from build123d import *

# Parameters (mm, degrees)
F0_W     = 30
F0_H     = 45
F1_DEPTH = 2
F2_W     = 30
F2_H     = 2
F2_H_2   = 5.5
F3_DEPTH = 2
F6_DEPTH = 25
F7_W     = 8
F7_H     = 11
F8_DEPTH = 2
F9_R     = 15
F10_R    = 5
F11_R    = 0.99999


# Not quite as in the source:
# - a fillet or chamfer is up to 0.001 mm smaller than in the source, because OpenCascade refuses the exact size
# - ends of sketch curves that miss each other by under 0.0002 mm in the source are joined


with BuildPart() as f1:
    # F0 (on Top) → F1 (new body)
    with BuildSketch(Plane.XY):
        with Locations((-15, -22.5)):
            Rectangle(F0_W, F0_H)
        with BuildLine():
            ThreePointArc((-27.75, -5), (-26, -3.25), (-24.25, -5))
            Line((-24.25, -5), (-24.25, -15))
            ThreePointArc((-24.25, -15), (-26, -16.75), (-27.75, -15))
            Line((-27.75, -15), (-27.75, -5))
        make_face(mode=Mode.SUBTRACT)
        with BuildLine():
            Line((-2.25, -15), (-2.25, -25))
            ThreePointArc((-2.25, -25), (-4, -26.75), (-5.75, -25))
            Line((-5.75, -25), (-5.75, -15))
            ThreePointArc((-5.75, -15), (-4, -13.25), (-2.25, -15))
        make_face(mode=Mode.SUBTRACT)
    extrude(amount=F1_DEPTH)

    # F2 (on face) → F3 (join)
    with BuildSketch(Plane.XZ.offset(45)):
        with Locations((-15, 1)):
            Rectangle(F2_W, F2_H)
        with Locations((-15, 4.75)):
            Rectangle(F2_W, F2_H_2)
    extrude(amount=F3_DEPTH)

    # F4: F1 across face


with BuildPart() as f1_1:
    add(f1.part)
    add(f1.part.mirror(Plane(origin=(-15, -46, 7.5), x_dir=(1, 0, 0), z_dir=(0, 0, 1))))

    # F5 (on face) → F6 (cut)
    with BuildSketch(Plane(origin=(0, -45, 0), x_dir=(-1, 0, 0), z_dir=(0, 1, 0))):
        with BuildLine():
            ThreePointArc((5.1587387914, 9.2572143), (3.4087387914, 7.5072143), (5.1587387913, 5.7572143))
            Line((5.1587387913, 5.7572143), (25.0000000102, 5.7500001157))
            ThreePointArc((25.0000000102, 5.7500001157), (26.7500000102, 7.5), (25.0000000102, 9.25))
            Line((25.0000000102, 9.25), (5.1587387914, 9.2572143))
        make_face()
    extrude(amount=-F6_DEPTH, mode=Mode.SUBTRACT)

    # F7 (on face) → F8 (join)
    with BuildSketch(Plane.YZ):
        Polygon((-37, 13), (-37, 15), (-47, 15), (-47, 0), (-37, 0), (-37, 2), (-45, 2), (-45, 13), align=None)
        with Locations((-41, 7.5)):
            Rectangle(F7_W, F7_H)
    extrude(amount=-F8_DEPTH)

    # F9
    f9_edges = [f1_1.edges().sort_by_distance(p)[0] for p in [
        (0, 0, 1),
        (0, 0, 14),
    ]]
    fillet(f9_edges, radius=F9_R)

    # F10
    f10_edges = [f1_1.edges().sort_by_distance(p)[0] for p in [
        (-30, 0, 14),
        (-30, 0, 1),
    ]]
    fillet(f10_edges, radius=F10_R)

    # F11 (radius 1 in the source; OpenCascade refuses exactly that, so slightly less here)
    f11_edges = [f1_1.edges().sort_by_distance(p)[0] for p in [
        (-2, -37, 7.5),
        (0, -37, 7.5),
    ]]
    fillet(f11_edges, radius=F11_R)


solid = f1_1.part
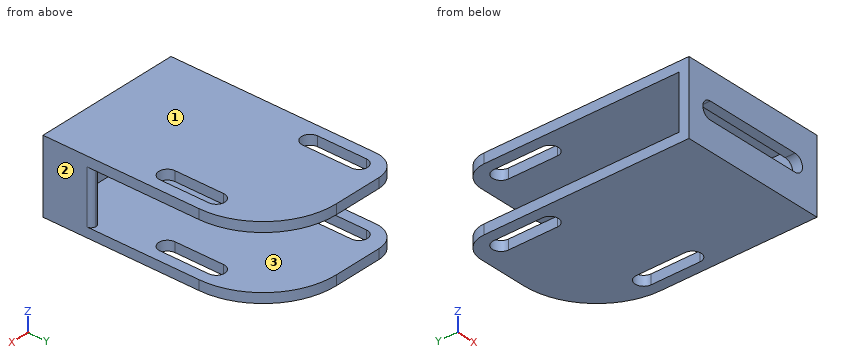
For this review, take the finished solid that the model builds, in its own axes (mm). Face numbers are marked on the shaded views. Give positions to 0.01 mm unless a question says otherwise; leave off trailing zeros. Loops run counter-clockwise (first coordinate to the right, second up) from the corner with the lowest first, then second, coordinate; pieces in that order, holes last. Notation, with made-up numbers: M -0.75,65 L 38.25,65 A29 cw 38.25,94 Z; hole C 22.25,19 d3. An arc over 180 degrees is marked long. Put each result on its own line as item: value. Start each with the question number.
(1) Wall thickness on L1, parallel to Z at x = -23, y = -13.5; L2, parallel to X at y = -24.5, z = 14.5; L3, parallel to Y at x = -23, z = 12: over which ranges is each line inside the solid? List them lowest first.
(2) Add section A-A, the plane y = -32.5. Write out the cut boundary in (x, z).
(3) The part is to be moulded in two halves that separate along Z. For the marked faces 1, 2 and 3, say which applies: +Z half, -Z half, draft (parallel to the pull), parting line (faces both ways), or undercut.
(4) Add section C-C, the plane y = -20.5. Write out the cut boundary in (x, z), then the cut area to 3 significant figures.
(5) For pin 1 (3.5 mm diameter, centred on x = -19.5, z = 5.5, fed in from +Y); pin 2 (0.6 mm diameter, centred on y = -9.5, z = 1, fed in from +X); pin 3 (7.5 mm diameter, centred on y = -41, z = 8.5, fed in from -X), all flat-tipped, find the tip position at first contact; note any pin that passes through.
Result:
1. L1: z = 0 to 2, 13 to 15
1. L2: x = -30 to -5.75, -2.25 to 0
1. L3: y = -47 to -45
2. outline: M -30,0 L 0,0 L 0,2 L -30,2 Z; M -30,13 L 0,13 L 0,15 L -30,15 Z
3. face 1: +Z half
3. face 2: draft
3. face 3: undercut
4. outline: M -30,0 L -5.75,0 L -5.75,2 L -30,2 Z; M -30,13 L -5.75,13 L -5.75,15 L -30,15 Z; M -2.25,0 L 0,0 L 0,2 L -2.25,2 Z; M -2.25,13 L 0,13 L 0,15 L -2.25,15 Z
4. area: 106 mm^2
5. pin 1: stops at y = -45
5. pin 2: stops at x = -0.93
5. pin 3: stops at x = -2
